```python
from build123d import *

# Parameters (mm, degrees)
SKETCH1_R           = 38
SKETCH1_R_2         = 2.55
BOSS_EXTRUDE1_DEPTH = 4.7


with BuildPart() as part:
    # Sketch1 → Boss-Extrude1 (new body)
    with BuildSketch(Plane(origin=(0, 0, 0), x_dir=(1, 0, 0), z_dir=(0, 1, 0))):
        with Locations(Location((0, 0, 0), (0, 0, 270))):
            Circle(SKETCH1_R)
        with Locations(Location((0, 0, 0), (0, 0, 270))):
            Circle(SKETCH1_R_2, mode=Mode.SUBTRACT)
        with BuildLine():
            Line((2.4, 8.979977728), (2.4, 25.624987805))
            ThreePointArc((2.4, 25.624987805), (3.110993227, 27.154190714), (4.738461538, 27.596140713))
            ThreePointArc((4.738461538, 27.596140713), (24.248711306, 14), (26.268189673, -9.694442289))
            ThreePointArc((26.268189673, -9.694442289), (25.071715591, -10.882896192), (23.391890411, -10.734032933))
            Line((23.391890411, -10.734032933), (8.976888838, -2.411527895))
            ThreePointArc((8.976888838, -2.411527895), (8.211845562, -1.620020671), (7.98151107, -0.54358167))
            ThreePointArc((7.98151107, -0.54358167), (6.92820323, 4), (3.52, 7.183982183))
            ThreePointArc((3.52, 7.183982183), (2.702943725, 7.921677204), (2.4, 8.979977728))
        make_face(mode=Mode.SUBTRACT)
        with BuildLine():
            Line((-2.4, 8.979977728), (-2.4, 25.624987805))
            ThreePointArc((-2.4, 25.624987805), (-3.110993227, 27.154190714), (-4.738461538, 27.596140713))
            ThreePointArc((-4.738461538, 27.596140713), (-24.248711306, 14), (-26.268189673, -9.694442289))
            ThreePointArc((-26.268189673, -9.694442289), (-25.071715591, -10.882896192), (-23.391890411, -10.734032933))
            Line((-23.391890411, -10.734032933), (-8.976888838, -2.411527895))
            ThreePointArc((-8.976888838, -2.411527895), (-8.211845562, -1.620020671), (-7.98151107, -0.54358167))
            ThreePointArc((-7.98151107, -0.54358167), (-6.92820323, 4), (-3.52, 7.183982183))
            ThreePointArc((-3.52, 7.183982183), (-2.702943725, 7.921677204), (-2.4, 8.979977728))
        make_face(mode=Mode.SUBTRACT)
        with BuildLine():
            Line((6.576888838, -6.568449833), (20.991890411, -14.890954872))
            ThreePointArc((20.991890411, -14.890954872), (21.960722365, -16.271294523), (21.529728135, -17.901698424))
            ThreePointArc((21.529728135, -17.901698424), (0, -28), (-21.529728135, -17.901698424))
            ThreePointArc((-21.529728135, -17.901698424), (-21.960722365, -16.271294523), (-20.991890411, -14.890954872))
            Line((-20.991890411, -14.890954872), (-6.576888838, -6.568449833))
            ThreePointArc((-6.576888838, -6.568449833), (-5.508901837, -6.301656533), (-4.46151107, -6.640400513))
            ThreePointArc((-4.46151107, -6.640400513), (0, -8), (4.46151107, -6.640400513))
            ThreePointArc((4.46151107, -6.640400513), (5.508901837, -6.301656533), (6.576888838, -6.568449833))
        make_face(mode=Mode.SUBTRACT)
    extrude(amount=BOSS_EXTRUDE1_DEPTH)


solid = part.part
```
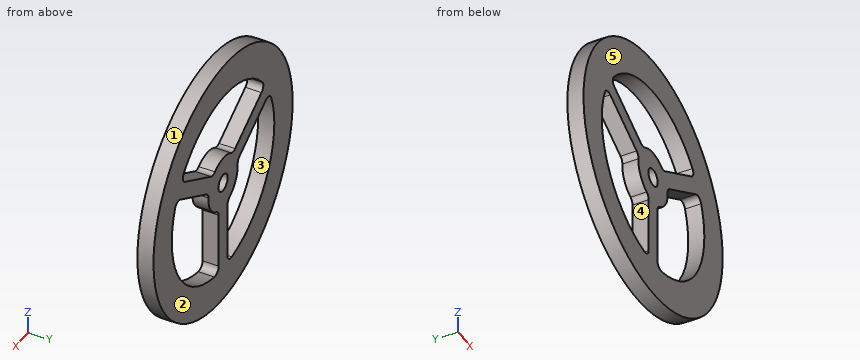
Source: CAD feature listing. Evaluate the final solid. Frame: model axes, mm. Face numbers are marked on the shaded views. A direction names the side the tool comes from. Round coordinates to 2 decimals unless told otherwise and drop trailing zeros. Order: outer loops, then holes, each group sorted by start corner. A loop starts at its lowest first (then second) coordinate and runs counter-clockwise, first axis right, second up. Notation, with made-up numbers: (33, -25.75) -> (84, -25.75) arc R21 ccw to (84, 12.25) -> close; hole circle Ø10 at (72.25, 72.25). An arc over 180 degrees is marked (long way). Use CSV: the item, a comma, the result in double quotes.
(1) Section A-A on x = 0. Return the cut outline in (y, z).
Report:
outline,"(0, -38) -> (4.7, -38) -> (4.7, -2.55) -> (0, -2.55) -> close; (0, 2.55) -> (4.7, 2.55) -> (4.7, 8) -> (0, 8) -> close; (0, 28) -> (4.7, 28) -> (4.7, 38) -> (0, 38) -> close"
(2) Access query for the marked faces 4 and 5. Directions: +Z, -Z, +X, -X, +Y, -Y. A direction counts if a zero-diameter tool reaches every point of the face in a straight line with its end or side. Return the directions, or none.
Report:
face 4,"+Y, -Y"
face 5,"+Z, -Z, +X, -X, -Y"
(3) Ray query, L1, parallel to X at y = 3.3, z = 0; L2, parallel to X at y = 0.85, z = -23.5; L3, parallel to Z at x = -21.5, y = 4.1. Return the intervals inside material, ascending.
Report:
L1,"-38 to -28, -8 to -2.55, 2.55 to 8, 28 to 38"
L2,"-29.86 to -15.22, -2.4 to 2.4, 15.22 to 29.86"
L3,"-31.33 to -17.94, 9.64 to 15.31, 17.94 to 31.33"
(4) Section C-C on z = -16. Return the cut outline in (x, y).
Report:
outline,"(-34.47, 0) -> (-22.98, 0) -> (-22.98, 4.7) -> (-34.47, 4.7) -> close; (-2.4, 0) -> (2.4, 0) -> (2.4, 4.7) -> (-2.4, 4.7) -> close; (22.98, 0) -> (34.47, 0) -> (34.47, 4.7) -> (22.98, 4.7) -> close"
(5) Pull-direction query (X, two-part tool) for the marked faces 1, 2 and 3; classes: +X half, -X half, draft (parallel to the pull), parting line (faces both ways), or undercut.
Report:
face 1,"parting line"
face 2,"draft"
face 3,"undercut"
(6) Section B-B on y = 3.5. Return the cut outline in (x, z), and give its area (3 significant figures).
Report:
outline,"circle Ø76 at (0, 0); hole (-26.27, 9.69) arc R28 ccw to (-4.74, -27.6) arc R2 ccw to (-2.4, -25.62) -> (-2.4, -8.98) arc R2 ccw to (-3.52, -7.18) arc R8 cw to (-7.98, 0.54) arc R2 ccw to (-8.98, 2.41) -> (-23.39, 10.73) arc R2 ccw to start; hole (-21.53, 17.9) arc R2 ccw to (-20.99, 14.89) -> (-6.58, 6.57) arc R2 ccw to (-4.46, 6.64) arc R8 cw to (4.46, 6.64) arc R2 ccw to (6.58, 6.57) -> (20.99, 14.89) arc R2 ccw to (21.53, 17.9) arc R28 ccw to start; hole circle Ø5.1 at (0, 0); hole (2.4, -25.62) arc R2 ccw to (4.74, -27.6) arc R28 ccw to (26.27, 9.69) arc R2 ccw to (23.39, 10.73) -> (8.98, 2.41) arc R2 ccw to (7.98, 0.54) arc R8 cw to (3.52, -7.18) arc R2 ccw to (2.4, -8.98) -> close"
area,"2,550 mm^2"
(7) First-contact query: pin 1 Ø12 at (x, z) = (-22.5, -7) entering from +Y; pin 2 Ø3 at (x, z) = (0, 0) entering from -Y; pin 3 Ø2.5 at (y, z) = (2, -18) entering from -X; pin 4 Ø2 at (y, z) = (1, -25) entering from +X. Flat tips, straight axial feed; report the tip coordinate or a pass-through.
Report:
pin 1,"y = 4.7"
pin 2,"through"
pin 3,"x = -34.11"
pin 4,"x = 29.46"
(8) Section D-D on z = 13. Return the cut outline in (x, y), and give its area (3 significant figures).
Report:
outline,"(-35.71, 0) -> (-17.72, 0) -> (-17.72, 4.7) -> (-35.71, 4.7) -> close; (17.72, 0) -> (35.71, 0) -> (35.71, 4.7) -> (17.72, 4.7) -> close"
area,"169 mm^2"
